Input: part model. Units: mm. Frame: model coordinates. Face numbers are marked on the shaded views. A direction names the side the tool comes from. Round coordinates to 2 decimals unless told otherwise and drop trailing zeros. Loops run counter-clockwise (first coordinate to the right, second up) from the corner with the lowest first, then second, coordinate; pieces in that order, holes last. Notation, with made-up numbers: M 35,82 L 48,82 A17 cw 48,106 Z; hole C 25.25,-4.5 d1. An arc over 180 degrees is marked long. Return JSON: item names as keys, results as strings. Group by question number.
1) Mould query, pull axis X, two halves, no side actions, for the marked faces 1, 2 and 3. Classes: +X half, -X half, draft (parallel to the pull), parting line (faces both ways), or undercut.
2) Section C-C (x = 33.25). Output: boundary loops of the cut face in (y, z), plus the area to 3 significant figures.
3) Section D-D (y = 29.5). Output: boundary loops of the cut face in (x, z).
4) Section A-A (y = 34). Output: boundary loops of the cut face in (x, z), plus the area to 3 significant figures.
5) Contact query for flat-ended pins moving along their axis: P1, Ø1, axis at y = 29, z = 91.5, coming from the +X side; P2, Ø2, axis at y = 29, z = 92, coming from the -X side; P3, Ø6, axis at x = 24.5, y = 31.5, coming from the +Z side. Output: stop coordinate, or through.
6) Access query for the marked faces 4, 5 and 6. Directions: +Z, -Z, +X, -X, +Y, -Y. A direction counts if a zero-diameter tool reaches every point of the face in a straight line with its end or side. Return the directions, or none.
7) Section B-B (z = 83.25). Output: boundary loops of the cut face in (x, y), plus the area to 3 significant figures.
8) Material intervals for line 1 (X direction, y = 32.5, z = 93.75); line 2 (X direction, y = 27.75, z = 90.75); line 3 (X direction, y = 30.5, z = 91), sorted ascending. Write a range as from..to.
from build123d import *

# Parameters (mm, degrees)
SKETCH037_R     = 2
PAD022_DEPTH    = 1.3
PAD023_DEPTH    = 2.7
SKETCH039_W     = 7
SKETCH039_H     = 2
PAD024_DEPTH    = 10
SKETCH040_R     = 2
POCKET010_DEPTH = 2
SKETCH041_W     = 8.5
SKETCH041_H     = 8.9
SKETCH041_R     = 2
PAD025_DEPTH    = 5
POCKET011_START = -0.9
POCKET011_DEPTH = 2.8
SKETCH043_W     = 4.5
SKETCH043_H     = 4.5
POCKET012_DEPTH = 1.301
FILLET005_R     = 2
FILLET006_R     = 1.7
FILLET007_R     = 3
SKETCH052_W     = 5
SKETCH052_H     = 8.5
POCKET017_DEPTH = 0.2
SKETCH053_W     = 0.4
SKETCH053_H     = 8.5
POCKET018_DEPTH = 8.7
PAD031_DEPTH    = 2


with BuildPart() as obj1:
    # Sketch037 → Pad022 (new body)
    with BuildSketch(Plane.XZ):
        Polygon((4.5, -4), (-4.3, -4), (-4.3, 3.24), (-14.8, 3.24), (-14.8, 7.49), (-14.8, 11.74), (-9.8, 11.74), (-9.8, 9.5), (2.5, 9.5), (2.5, 5), (4.5, 5), align=None)
        Circle(SKETCH037_R, mode=Mode.SUBTRACT)
    extrude(amount=PAD022_DEPTH)

    # Sketch038 (on Face14 of Pad022) → Pad023 (join)
    with BuildSketch(Plane.XZ.offset(1.3)):
        Polygon((-4.090897, 0), (-2.045448, -3.54282), (2.045448, -3.54282), (4.090897, 0), (2.045448, 3.54282), (-2.045448, 3.54282), align=None)
        Polygon((-3.290897, 0), (-1.645448, -2.85), (1.645448, -2.85), (3.290897, 0), (1.645448, 2.85), (-1.645448, 2.85), align=None, mode=Mode.SUBTRACT)
    extrude(amount=PAD023_DEPTH)

    # Sketch039 (on Face5 of Pad023) → Pad024 (join)
    with BuildSketch(Plane.XZ.offset(1.3)):
        with Locations((-5.5, 8.5)):
            Rectangle(SKETCH039_W, SKETCH039_H)
    extrude(amount=PAD024_DEPTH)

    # Sketch040 (on Face24 of Pad024) → Pocket010 (cut)
    with BuildSketch(Plane(origin=(0, 0, 9.5), x_dir=(-1, 0, 0), z_dir=(0, 0, 1))):
        with Locations((5.5, 7.7)):
            Circle(SKETCH040_R)
    extrude(amount=-POCKET010_DEPTH, mode=Mode.SUBTRACT)

    # Sketch041 (on Face6 of Pocket010) → Pad025 (join)
    with BuildSketch(Plane(origin=(-14.8, 0, 0), x_dir=(0, 0, -1), z_dir=(-1, 0, 0))):
        with Locations((-7.49, 5.75)):
            Rectangle(SKETCH041_W, SKETCH041_H)
        with Locations((-7.49, 6.8)):
            Circle(SKETCH041_R, mode=Mode.SUBTRACT)
    extrude(amount=-PAD025_DEPTH)

    # Sketch042 (on Face7 of Pad025) → Pocket011 (cut)
    with BuildSketch(Plane(origin=(-14.8, 0, 0), x_dir=(0, 0, -1), z_dir=(-1, 0, 0)).offset(POCKET011_START)):
        Polygon((-10.44, 8.503183), (-11.74, 8.503183), (-11.74, 10.2), (-3.24, 10.2), (-3.24, 8.503183), (-4.54, 8.503183), (-4.54, 5.096817), (-7.49, 3.393633), (-10.44, 5.096817), align=None)
    extrude(amount=-POCKET011_DEPTH, mode=Mode.SUBTRACT)

    # Sketch043 (on Face24 of Pocket011) → Pocket012 (cut, through all)
    with BuildSketch(Plane.XZ.offset(1.3)):
        with Locations((0.25, 7.25)):
            Rectangle(SKETCH043_W, SKETCH043_H)
    extrude(amount=-POCKET012_DEPTH, mode=Mode.SUBTRACT)

    # Fillet005
    fillet005_edges = [obj1.edges().sort_by_distance(p)[0] for p in [
        (-2, -0.65, 5),
        (4.5, -0.65, -4),
        (-4.3, -0.65, -4),
        (-4.3, -0.65, 3.24),
    ]]
    fillet(fillet005_edges, radius=FILLET005_R)

    # Fillet006
    fillet006_edges = [obj1.edges().sort_by_distance(p)[0] for p in [
        (4.5, -0.65, 5),
    ]]
    fillet(fillet006_edges, radius=FILLET006_R)

    # Fillet007
    fillet007_edges = [obj1.edges().sort_by_distance(p)[0] for p in [
        (-9, -11.3, 8.5),
        (-2, -11.3, 8.5),
    ]]
    fillet(fillet007_edges, radius=FILLET007_R)

    # Sketch052 (on Face43 of Fillet007) → Pocket017 (cut)
    with BuildSketch(Plane.XZ.offset(10.2)):
        with Locations((-12.3, 7.49)):
            Rectangle(SKETCH052_W, SKETCH052_H)
    extrude(amount=-POCKET017_DEPTH, mode=Mode.SUBTRACT)

    # Sketch053 (on Face37 of Pocket017) → Pocket018 (cut)
    with BuildSketch(Plane.XZ.offset(10)):
        with Locations((-10, 7.49)):
            Rectangle(SKETCH053_W, SKETCH053_H)
    extrude(amount=-POCKET018_DEPTH, mode=Mode.SUBTRACT)

    # Sketch055 (on Face2 of Pocket018) → Pad031 (join)
    with BuildSketch(Plane(origin=(0, 0, 7.5), x_dir=(1, 0, 0), z_dir=(0, 0, -1))):
        Polygon((-8.45, 9.403183), (-8.45, 5.996817), (-5.5, 4.293633), (-2.55, 5.996817), (-2.55, 9.403183), (-2, 9.403183), (-2, 1.3), (-9, 1.3), (-9, 9.403183), align=None)
    extrude(amount=PAD031_DEPTH)


with BuildPart() as obj1_1:
    # Body024 placement: moved
    add(obj1.part.moved(Location((-21.5, 36.8, 85))))


with BuildPart() as part_mirroring001:
    # Part__Mirroring001: instance of obj1
    add(obj1_1.part.mirror(Plane(origin=(0, 0, 0), x_dir=(0, -1, 0), z_dir=(1, 0, 0))))


solid = part_mirroring001.part
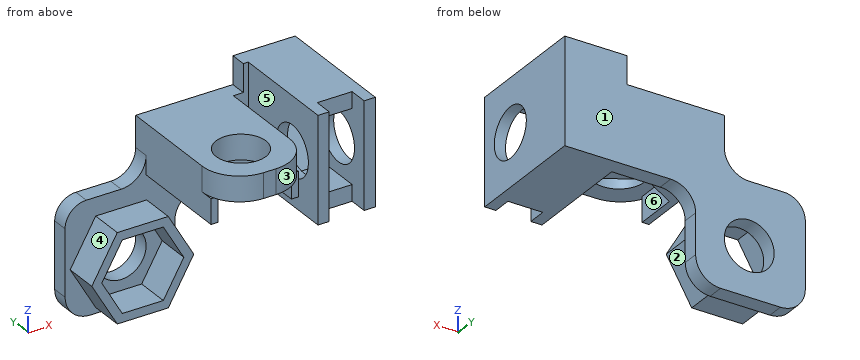
Returned:
{
 "1": {"face 1": "draft", "face 2": "+X half", "face 3": "undercut"},
 "2": {"outline": "M 28.3,88.24 L 36.8,88.24 L 36.8,96.74 L 28.3,96.74 L 28.3,95.44 L 31.7,95.44 L 33.41,92.49 L 31.7,89.54 L 28.3,89.54 Z", "area": "47.2 mm^2"},
 "3": {"outline": "M 23.5,90.5 L 24.05,90.5 L 24.05,92.5 L 25.04,92.5 L 25.04,94.5 L 23.5,94.5 Z; M 28.96,92.5 L 29.95,92.5 L 29.95,90.5 L 30.5,90.5 L 30.5,94.5 L 28.96,94.5 Z; M 31.7,88.24 L 36.3,88.24 L 36.3,90.55 L 35.4,90.55 L 35.4,89.54 L 32.6,89.54 L 32.6,90.55 L 31.7,90.55 Z; M 31.7,94.43 L 32.6,94.43 L 32.6,95.44 L 35.4,95.44 L 35.4,94.43 L 36.3,94.43 L 36.3,96.74 L 31.7,96.74 Z"},
 "4": {"outline": "M 17.41,85 L 19.45,81.46 L 23.55,81.46 L 25.59,85 L 23.55,88.54 L 19.45,88.54 Z; M 23.5,90.5 L 30.5,90.5 L 30.5,94.5 L 23.5,94.5 Z; M 31.7,88.24 L 36.3,88.24 L 36.3,96.74 L 31.7,96.74 Z; hole M 18.21,85 L 19.85,82.15 L 23.15,82.15 L 24.79,85 L 23.15,87.85 L 19.85,87.85 Z", "area": "82.4 mm^2"},
 "5": {"P1": "stops at x = 30.5", "P2": "stops at x = 23.5", "P3": "stops at z = 94.5"},
 "6": {"face 4": "+Z, -X, -Y", "face 5": "+Z, -Z, -Y", "face 6": "-Z, -Y"},
 "7": {"outline": "M 17,35.5 L 18.42,35.5 L 18.42,32.8 L 19.22,32.8 L 19.22,35.5 L 20.53,35.5 L 20.53,36.8 L 17,36.8 Z; M 22.47,35.5 L 23.78,35.5 L 23.78,32.8 L 24.58,32.8 L 24.58,35.5 L 25.8,35.5 L 25.8,36.8 L 22.47,36.8 Z", "area": "13.2 mm^2"},
 "8": {"line 1": "x = 23.5..30.5, 31.7..32.6, 35.4..36.3", "line 2": "x = 23.5..24.05, 29.95..30.5, 31.7..32.6, 35.4..36.3", "line 3": "x = 23.5..24.05, 29.95..30.5"}
}
